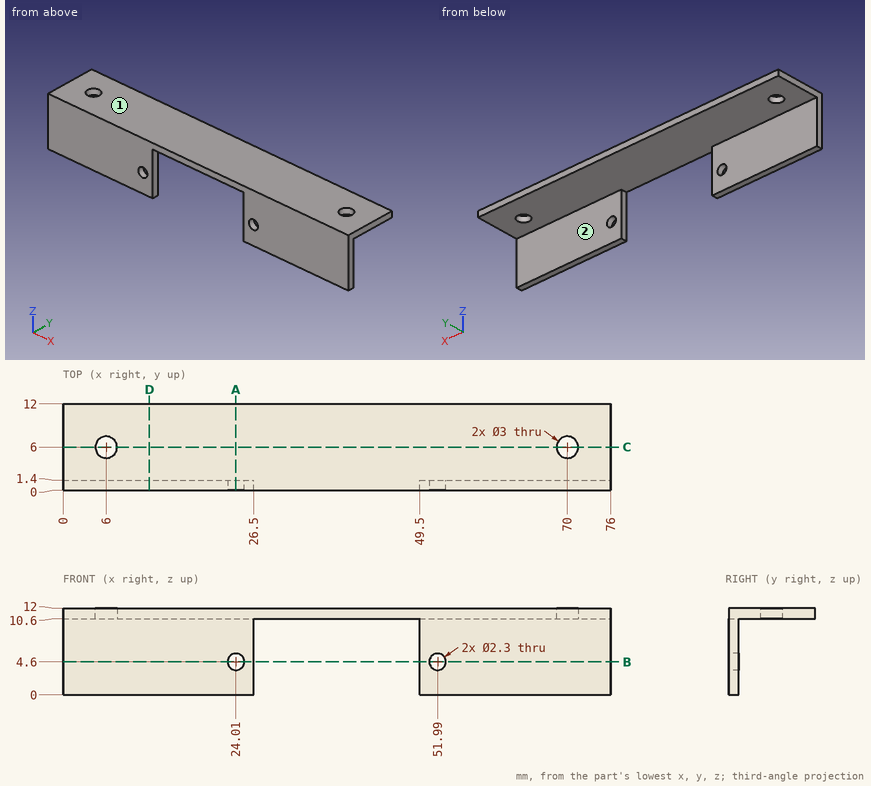
For this review, use the dimensioned drawing (mm, ordinates from the lowest corner) and the shaded views. A direction names the side the tool comes from. Round coordinates to 2 decimals unless told otherwise and drop trailing zeros. Order: outer loops, then holes, each group sorted by start corner. A loop starts at its lowest first (then second) coordinate and runs counter-clockwise, first axis right, second up. Notation, with made-up numbers: (31.5, 78) -> (68.5, 78) arc R12 ccw to (68.5, 89) -> close; hole circle Ø6 at (63.25, 51). An arc over 180 degrees is marked (long way). One line per item, written item: value. Start each with the question number.
Q1. Take a section at D-D (x = 12). Write out the cut boundary in (y, z), and give its area (3 significant figures).
Q2. Take a section at C-C (y = 6). Write out the cut boundary in (x, z).
Q3. Take a section at B-B (z = 4.6). Write out the cut boundary in (x, y).
Q4. Take a section at A-A (x = 24.01). Write out the cut boundary in (y, z), and give its area (3 significant figures).
Q5. Machinability: for the marked faces 1 and 2, which of the approach directions +Z, -Z, +X, -X, +Y, -Y give a long, thin tool a straight path to every point of the face, cutting with its end or side? Answer none if there is none.
Q6. Clearance check with flat-ended pins moving along their axes: pin 1 Ø6 at (x, y) = (41, 4.5) entering from -Z; pin 2 Ø3 at (x, z) = (19.5, 3.5) entering from +Y. State where each tip first meets the part, or that it passes through.
Q7. Wall thickness on line 1 (Y direction, x = 70, z = 10.95); line 2 (Z direction, x = 51.99, y = 0.95); line 3 (Z direction, x = 60, y = 4.75): over which ranges is each line inside the solid? List them lowest first.
Reported:
1. outline: (0, 0) -> (1.4, 0) -> (1.4, 10.6) -> (12, 10.6) -> (12, 12) -> (0, 12) -> close
1. area: 31.6 mm2
2. outline: (0, 10.6) -> (4.5, 10.6) -> (4.5, 12) -> (0, 12) -> close; (7.5, 10.6) -> (68.5, 10.6) -> (68.5, 12) -> (7.5, 12) -> close; (71.5, 10.6) -> (76, 10.6) -> (76, 12) -> (71.5, 12) -> close
3. outline: (0, 0) -> (22.86, 0) -> (22.86, 1.4) -> (0, 1.4) -> close; (25.16, 0) -> (26.5, 0) -> (26.5, 1.4) -> (25.16, 1.4) -> close; (49.5, 0) -> (50.84, 0) -> (50.84, 1.4) -> (49.5, 1.4) -> close; (53.14, 0) -> (76, 0) -> (76, 1.4) -> (53.14, 1.4) -> close
4. outline: (0, 0) -> (1.4, 0) -> (1.4, 3.45) -> (0, 3.45) -> close; (0, 5.75) -> (1.4, 5.75) -> (1.4, 10.6) -> (12, 10.6) -> (12, 12) -> (0, 12) -> close
4. area: 28.4 mm2
5. face 1: +Z, +X, -X, +Y, -Y
5. face 2: -Z, +X, -X, +Y
6. pin 1: stops at z = 10.6
6. pin 2: stops at y = 1.4
7. line 1: y = 0 to 4.5, 7.5 to 12
7. line 2: z = 0 to 3.45, 5.75 to 12
7. line 3: z = 10.6 to 12
